Autodesk Inventor part; units mm, degrees
ref_plane "YZ Plane" through (0, 0, 0) normal (1, 0, 0) x (0, 1, 0)
ref_plane "XZ Plane" through (0, 0, 0) normal (0, 1, 0) x (-1, 0, 0)
ref_plane "XY Plane" through (0, 0, 0) normal (0, 0, 1) x (1, 0, 0)
sketch "Sketch1" plane through (0, 0, 0) normal (0, 0, 1) x (1, 0, 0)
  arc A0 (-5.9942, 51.8019) -> (-3.0058, 51.8019) centre (-4.5, 55) ccw
  line L0 (8.4999, 69.9999) -> (0, 69.9999)
  line L1 (-9, 40.0001) -> (-17.4999, 40.0001)
  line L2 (10.4999, 0) -> (10.4999, 69.9999)
  line L3 (-19.4999, 0) -> (-19.4999, 69.9999)
  line L4 (-19.4999, 69.9999) -> (10.4999, 69.9999)
  line L5 (10.4999, 69.9999) -> (10.4999, 40.0001)
  line L6 (10.4999, 40.0001) -> (-19.4999, 40.0001)
  line L7 (-19.4999, 40.0001) -> (-19.4999, 69.9999)
  circle A1 centre (-4.5, 55) radius 3.75
  point P0 (0, 0)
  dimension "d0" = 29.9999
  dimension "d1" = 29.9999
  dimension "d2" = 14.9999
  dimension "d3" = 7.5
extrude "Plate1" add sketch "Sketch1" along normal blind 2
equation "\"BendRadius\" = Thickness"
equation "\"BendReliefWidth\" = Thickness"
equation "\"BendReliefDepth\" = 0.5 * Thickness"
equation "\"CornerReliefSize\" = 4 * Thickness"
equation "\"MinimumRemnant\" = 2 * Thickness"
equation "\"TransitionRadius\" = BendRadius"
equation "\"JacobiRadiusSize\" = BendRadius"
equation "\"GapSize\" = Thickness"
equation "\"d4\" = BendRadius"
properties part number "gabarito-30" material "Wood (Oak)"
For this review, take the finished solid that the model builds, in its own axes (mm). Coordinates: 2 decimals unless noted, no trailing zeros. Order: outer loops, then holes, each group sorted by start corner. A loop starts at its lowest first (then second) coordinate and runs counter-clockwise, first axis right, second up. Notation, with made-up numbers: (47, 40.25) -> (78, 40.25) arc R20 cw to (78, 73.25) -> close; hole circle Ø4 at (-6.75, -36.5). An arc over 180 degrees is marked (long way). Return JSON: item names as keys, results as strings.
1. For pin 1 Ø10 at (x, y) = (-10, 60) entering from -Z, flat-tipped, find the tip position at first contact; note if it passes through.
Answer block:
{"pin 1": "z = 0"}
2. The part is to be moulded in two halves that separate along X. For faces 1 (the flat face through (-19.5, 55, 1)), 2 (the flat face through (-8, 59, 0)), 3 (the flat face through (10.5, 55, 1)), 4 (the cylindrical face through (-5.31, 58.66, 0.99)), say which applies: +X half, -X half, draft (parallel to the pull), parting line (faces both ways), or undercut.
Answer block:
{"face 1": "-X half", "face 2": "draft", "face 3": "+X half", "face 4": "undercut"}
3. We need section B-B on x = -4.5. Write out the cut boundary in (y, z).
Answer block:
{"outline": "(40, 0) -> (51.25, 0) -> (51.25, 2) -> (40, 2) -> close; (58.75, 0) -> (70, 0) -> (70, 2) -> (58.75, 2) -> close"}
4. We need section A-A on y = 58. Write out the cut boundary in (x, z).
Answer block:
{"outline": "(-19.5, 0) -> (-6.75, 0) -> (-6.75, 2) -> (-19.5, 2) -> close; (-2.25, 0) -> (10.5, 0) -> (10.5, 2) -> (-2.25, 2) -> close"}
5. For line 1 (Y direction, x = -4.5, z = 0.65); line 2 (Y direction, x = -2, z = 0.85); line 3 (X direction, y = 56, z = 1.9), list the stretches that pass through material, from the lowest coordinate up. Write a range as from..to.
Answer block:
{"line 1": "40..51.25, 58.75..70", "line 2": "40..52.2, 57.8..70", "line 3": "-19.5..-8.11, -0.89..10.5"}
6. We need section C-C on z = 1.4. Write out the cut boundary in (x, y), and give its area (3 significant figures).
Answer block:
{"outline": "(-19.5, 40) -> (10.5, 40) -> (10.5, 70) -> (-19.5, 70) -> close; hole circle Ø7.5 at (-4.5, 55)", "area": "856 mm²"}
